Here's the drawing with two shaded views (mm, measured from the low corner). I have some questions. A direction names the side the tool comes from. Coordinates: 2 decimals unless noted, no trailing zeros. Loops run counter-clockwise (first coordinate to the right, second up) from the corner with the lowest first, then second, coordinate; pieces in that order, holes last. Notation, with made-up numbers: (-18, 83.25) -> (-14, 83.25) arc R33 ccw to (-14, 112.25) -> close; hole circle Ø11 at (29, 28). An arc over 180 degrees is marked (long way). Answer as a JSON object with one key per item and string values. Group by question number.
Q1. I want a section at D-D on y = 1.75. Write out the boundary of the cut face in (x, z).
Q2. On a 3-axis mill with a long thin cutter (end or side, diameter ignored), from which of +Z, -Z, +X, -X, +Y, -Y can I reach the whole of each face in a straight line? I mean the marked faces 1 and 2. Say none if no direction works.
Q3. I need wall thicknesses on line 1 (Z direction, x = 4, y = 1.6); line 2 (Y direction, x = 2, z = 7.75); line 3 (X direction, y = 7, z = 0.75). Which ranges of each line are inside material? Lowest first, please.
Q4. Thinking about a two-plate mould opening in Y: for the marked faces 3, 4, 5 and 6, which applies, released by +Y, released by -Y, zero draft, split by the parting line, or undercut?
Q5. I want a section at A-A on z = 4.5. Write out the boundary of the cut face in (x, y), then the cut area to 3 significant figures.
Q6. I want a section at B-B on x = 4. Write out the boundary of the cut face in (y, z).
Q7. I'm going to push flat-ended pins straight in: pin 1 (1.5 mm diameter, centred on x = 1, y = 3, fed in from -Z); pin 2 (1.6 mm diameter, centred on x = 4, z = 5, fed in from -Y). Where does each tip first touch, or does it pass through?
Q8. I want a section at C-C on x = 2. Write out the boundary of the cut face in (y, z).
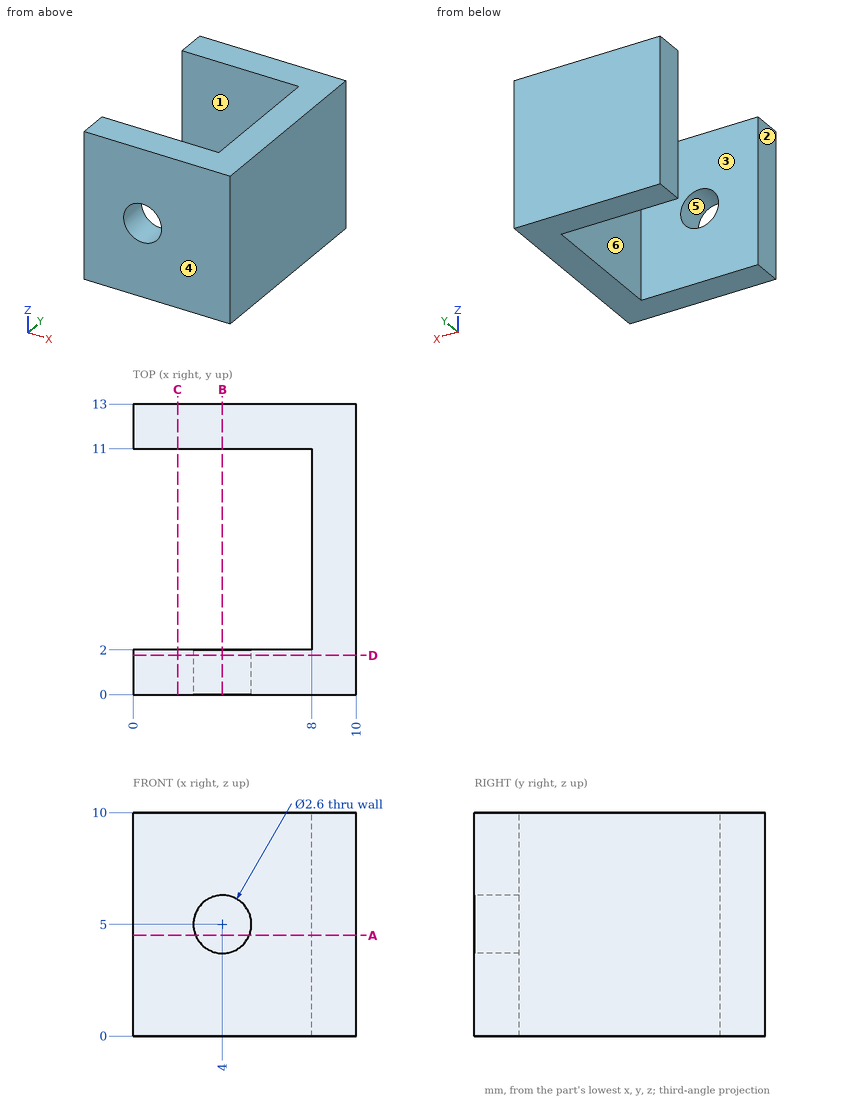
Result set:
{
 "1": {"outline": "(0, 0) -> (10, 0) -> (10, 10) -> (0, 10) -> close; hole circle Ø2.6 at (4, 5)"},
 "2": {"face 1": "+Z, -Z, -X", "face 2": "+Z, -Z, -X, +Y, -Y"},
 "3": {"line 1": "z = 0 to 3.7, 6.3 to 10", "line 2": "y = 0 to 2, 11 to 13", "line 3": "x = 8 to 10"},
 "4": {"face 3": "undercut", "face 4": "released by -Y", "face 5": "zero draft", "face 6": "undercut"},
 "5": {"outline": "(0, 0) -> (2.8, 0) -> (2.8, 2) -> (0, 2) -> close; (0, 11) -> (8, 11) -> (8, 2) -> (5.2, 2) -> (5.2, 0) -> (10, 0) -> (10, 13) -> (0, 13) -> close", "area": "53.2 mm²"},
 "6": {"outline": "(0, 0) -> (2, 0) -> (2, 3.7) -> (0, 3.7) -> close; (0, 6.3) -> (2, 6.3) -> (2, 10) -> (0, 10) -> close; (11, 0) -> (13, 0) -> (13, 10) -> (11, 10) -> close"},
 "7": {"pin 1": "passes through", "pin 2": "stops at y = 11"},
 "8": {"outline": "(0, 0) -> (2, 0) -> (2, 10) -> (0, 10) -> close; (11, 0) -> (13, 0) -> (13, 10) -> (11, 10) -> close"}
}
